Autodesk Inventor part; units mm, degrees
ref_plane "YZ Plane" through (0, 0, 0) normal (1, 0, 0) x (0, 1, 0)
ref_plane "XZ Plane" through (0, 0, 0) normal (0, 1, 0) x (-1, 0, 0)
ref_plane "XY Plane" through (0, 0, 0) normal (0, 0, 1) x (1, 0, 0)
sketch "Sketch1" plane through (0, 0, 0) normal (0, 1, 0) x (-1, 0, 0)
  line L0 (0, 20.9385) -> (0, -224.0391)
  ellipse E0 centre (275, -2.2065) end of major axis (0, -2.2065) minor radius 200 (275, 197.7935) -> (0, -2.2065) ccw
  ellipse E1 centre (275, -2.2065) end of major axis (40, -2.2065) minor radius 100 (275, 97.7935) -> (40, -2.2065) ccw
  line L1 (0, -2.2065) -> (40, -2.2065)
  line L2 (30.5, -2.2065) -> (9.5, -2.2065)
  line L3 (9.5, -2.2065) -> (9.5, 2.7935)
  line L4 (9.5, 2.7935) -> (30.5, 2.7935)
  line L5 (30.5, 2.7935) -> (30.5, -2.2065)
  line L6 (0, -2.2065) -> (9.5, -2.2065)
  line L7 (9.5, -2.2065) -> (9.5, -27.2065)
  line L8 (9.5, -27.2065) -> (0, -27.2065)
  line L9 (0, -27.2065) -> (0, -2.2065)
  line L10 (30.5, -2.2065) -> (40, -2.2065)
  line L11 (40, -2.2065) -> (40, -27.2065)
  line L12 (40, -27.2065) -> (30.5, -27.2065)
  line L13 (30.5, -27.2065) -> (30.5, -2.2065)
  line L14 (275, -2.2065) -> (275, 197.7935)
  line L15 (550, 20.9385) -> (550, -224.0391)
  ellipse E2 centre (275, -2.2065) end of major axis (550, -2.2065) minor radius 200 (550, -2.2065) -> (275, 197.7935) ccw
  ellipse E3 centre (275, -2.2065) end of major axis (510, -2.2065) minor radius 100 (510, -2.2065) -> (275, 97.7935) ccw
  line L16 (550, -2.2065) -> (510, -2.2065)
  line L17 (519.5, -2.2065) -> (540.5, -2.2065)
  line L18 (540.5, -2.2065) -> (540.5, 2.7935)
  line L19 (540.5, 2.7935) -> (519.5, 2.7935)
  line L20 (519.5, 2.7935) -> (519.5, -2.2065)
  line L21 (550, -2.2065) -> (540.5, -2.2065)
  line L22 (540.5, -2.2065) -> (540.5, -27.2065)
  line L23 (540.5, -27.2065) -> (550, -27.2065)
  line L24 (550, -27.2065) -> (550, -2.2065)
  line L25 (519.5, -2.2065) -> (510, -2.2065)
  line L26 (510, -2.2065) -> (510, -27.2065)
  line L27 (510, -27.2065) -> (519.5, -27.2065)
  line L28 (519.5, -27.2065) -> (519.5, -2.2065)
  point P0 (40, -2.2065)
  point P1 (0, -27.2065)
  dimension "d7" = 275
  dimension "d8" = 235
  dimension "d9" = 100
  dimension "d10" = 200
  dimension "d13" = 21
  dimension "d14" = 9.5
  dimension "d15" = 5
  dimension "d16" = 9.5
  dimension "d17" = 9.5
  dimension "d18" = 25
  dimension "d19" = 25
  dimension "d20" = 30
extrude "Extrusion1" add sketch "Sketch1" along normal blind 100 contours L1 L7 L8 L0 | E0 L14 E1 L1 L5 L4 L3 | E2 L16 L18 L19 L20 E3 L14 | L15 L23 L22 L16 | L1 L11 L12 L13 | L16 L28 L27 L26
sketch "Sketch2" plane through (0, 100, 0) normal (0, 1, 0) x (1, 0, 0)
  line L0 (-234, -145) -> (-316, -145)
  line L1 (-316, -145) -> (-316, -247)
  line L2 (-316, -247) -> (-234, -247)
  line L3 (-234, -247) -> (-234, -145)
  point P0 (0, 0)
  point P1 (-275, -145)
  dimension "d21" = 102
  dimension "d22" = 82
  dimension "d23" = 234
  dimension "d24" = 145
extrude "Extrusion2" cut sketch "Sketch2" against normal blind 300
sketch "Sketch3" plane through (-550, 0, -27.2065) normal (-1, 0, 0) x (0, 0, 1)
  circle A0 centre (15, 15) radius 5.5
  circle A1 centre (15, 85) radius 5.5
  line L0 (0, 0) -> (0, 100)
  line L1 (0, 0) -> (25, 0)
  line L2 (0, 100) -> (25, 100)
  point P0 (27.2065, 0)
  dimension "d27" = 11
  dimension "d28" = 11
  dimension "d29" = 15
  dimension "d30" = 15
  dimension "d31" = 15
  dimension "d32" = 15
extrude "Extrusion3" cut sketch "Sketch3" against normal blind 700
properties part number "CurvedSeatHolder" material "PET Plastic"
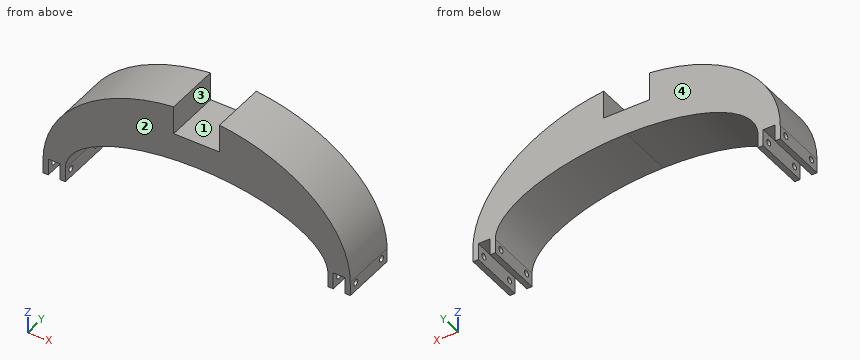
Source: CAD feature listing. Evaluate the final solid. Frame: model axes, mm. Face numbers are marked on the shaded views. A direction names the side the tool comes from. Coordinates: 2 decimals unless noted, no trailing zeros. Use a Markdown table: item, result.
1) Section A-A, the plane y = 15. Give the number of separate pieces and of enclosed holes in the cut face, then the cut area to 3 significant figures.
Conclusion:
| item | result |
|---|---|
| separate pieces | 5 |
| enclosed holes | 0 |
| area | 45,500 mm^2 |
2) First-contact query: pin 1 Ø17 at (x, y) = (-528.5, 38) entering from -Z; pin 2 Ø1.5 at (x, y) = (-284, 48.5) entering from -Z; pin 3 Ø6 at (x, y) = (-84.5, 16.5) entering from +Z. Flat tips, straight axial feed; report the tip coordinate or a pass-through.
Conclusion:
| item | result |
|---|---|
| pin 1 | stops at z = 2.79 |
| pin 2 | stops at z = 97.71 |
| pin 3 | stops at z = 144.1 |
3) Mould query, pull axis X, two halves, no side actions, for the marked faces 3 and 4. Classes: pulls with the +X half, pulls with the -X half, needs draft (parallel to the pull), parting line crosses it, or undercut.
Conclusion:
| item | result |
|---|---|
| face 3 | undercut |
| face 4 | needs draft |
4) Reachability of the marked faces 1 and 2 from +Z, -Z, +X, -X, +Y, -Y: full face, straight path, thin tool, end or side. Return the list, or none.
Conclusion:
| item | result |
|---|---|
| face 1 | +Z, +Y, -Y |
| face 2 | +Z, -Z, +X, -X, -Y |
5) Ray query, L1, parallel to X at y = 5.5, z = -17; L2, parallel to X at y = 46.5, z = 69; L3, parallel to X at y = 94, z = 158.5. Return the intervals inside material, ascending.
Conclusion:
| item | result |
|---|---|
| L1 | x = -550 to -540.5, -519.5 to -510, -40 to -30.5, -9.5 to 0 |
| L2 | x = -531.98 to -440, -110 to -18.02 |
| L3 | x = -438.7 to -316, -234 to -111.3 |
